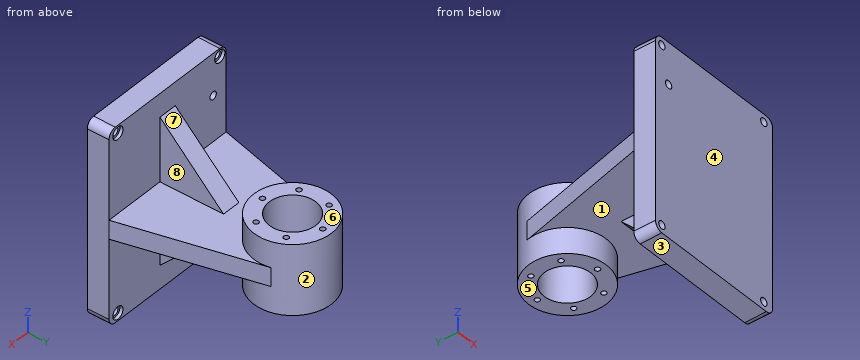
```python
from build123d import *

# Parameters (mm, degrees)
SKETCH_1_R                   = 25
SKETCH_1_R_2                 = 15
EXTRUDE_1_DEPTH              = 22.5
SKETCH_2_W                   = 92
SKETCH_2_H                   = 14
EXTRUDE_2_DEPTH              = 62
EXTRUDE_3_DEPTH              = 6
RIB_1_REACH                  = 123.639
SKETCH_5_WALL_W              = 303.26037525
SKETCH_5_WALL_H              = 12
FILLET_1_R                   = 5
HOLE_WIZARD_M4_2_D           = 5
HOLE_WIZARD_M4_2_CBORE_D     = 8
HOLE_WIZARD_M4_2_CBORE_DEPTH = 2
PATTERN_LINEAR_1_COUNT       = 2
PATTERN_LINEAR_1_PITCH       = 80
PATTERN_LINEAR_1_COUNT_DIR2  = 2
PATTERN_LINEAR_1_PITCH_DIR2  = 114
HOLE_WIZARD_M6_1_D           = 5
PATTERN_CIRCULAR_1_COUNT     = 6


with BuildPart() as part:
    # Sketch 1 → Extrude 1 (new, symmetric)
    with BuildSketch(Plane.XY):
        with Locations(Location((0, 0.57540869, 0), (0, 0, 180))):
            Circle(SKETCH_1_R)
        with Locations(Location((0, 0.57540869, 0), (0, 0, 180))):
            Circle(SKETCH_1_R_2, mode=Mode.SUBTRACT)
    extrude(amount=EXTRUDE_1_DEPTH, both=True)



with BuildPart() as body_2:
    # Sketch 2 → Extrude 2 (new, symmetric)
    with BuildSketch(Plane.XY):
        with Locations((0, -87)):
            Rectangle(SKETCH_2_W, SKETCH_2_H)
    extrude(amount=EXTRUDE_2_DEPTH, both=True)


with BuildPart() as part_1:
    add(part.part)

    add(body_2.part)  # Extrude 3 merges body 2
    # Sketch 4 → Extrude 3 (add, symmetric)
    with BuildSketch(Plane.XY):
        with BuildLine():
            Line((-24.247840613, 6.661641155), (-46, -80))
            Line((-46, -80), (46, -80))
            Line((46, -80), (24.247840613, 6.661641155))
            ThreePointArc((24.247840613, 6.661641155), (0, -24.42459131), (-24.247840613, 6.661641155))
        make_face()
    extrude(amount=EXTRUDE_3_DEPTH, both=True)

    # Sketch 5 wall → Rib 1 (add, up to next)
    with BuildSketch(Plane(origin=(0, -59.5, 26.5), x_dir=(0, 0.707106781187, -0.707106781187), z_dir=(0, 0.707106781187, 0.707106781187)), mode=Mode.PRIVATE) as rib_1_sk1:
        Rectangle(SKETCH_5_WALL_W, SKETCH_5_WALL_H)
    rib_1_tool1 = extrude(rib_1_sk1.sketch, amount=-RIB_1_REACH, mode=Mode.PRIVATE) - part_1.part
    rib_1 = rib_1_tool1.solids().sort_by_distance((0, -59.5, 26.5))[0]
    add(rib_1)

    # Mirror 1: Rib 1 across plane
    add(rib_1.mirror(Plane.XY))

    # Fillet 1
    fillet_1_edges = [part_1.edges().sort_by_distance(p)[0] for p in [
        (-46, -87, -62),
        (46, -87, 62),
        (-46, -87, 62),
        (46, -87, -62),
    ]]
    fillet(fillet_1_edges, radius=FILLET_1_R)

    # Hole Wizard M4 _ _ _ _ _2 (through all)
    with Locations(Plane(origin=(-41, -80, 57), x_dir=(0, 0, 1), z_dir=(0, 1, 0))):
        with Locations((0, 0)):
            hole_wizard_m4_2 = CounterBoreHole(HOLE_WIZARD_M4_2_D / 2, HOLE_WIZARD_M4_2_CBORE_D / 2, HOLE_WIZARD_M4_2_CBORE_DEPTH)

    # Pattern Linear 1: Hole Wizard M4 _ _ _ _ _2 2 × 2
    with Locations(*[(i * PATTERN_LINEAR_1_PITCH, 0, -j * PATTERN_LINEAR_1_PITCH_DIR2) for i in range(PATTERN_LINEAR_1_COUNT) for j in range(PATTERN_LINEAR_1_COUNT_DIR2) if (i, j) != (0, 0)]):
        add(hole_wizard_m4_2, mode=Mode.SUBTRACT)

    # Hole Wizard M6 _ _1 (through all)
    with Locations(Plane(origin=(-35.723311544, -80, 35.243458723), x_dir=(0, 0, 1), z_dir=(0, 1, 0))):
        with Locations((0, 0)):
            Hole(HOLE_WIZARD_M6_1_D / 2)

    # Sketch 21 → Hole Wizard M4 _ _1 (revolve, cut)
    with BuildSketch(Plane(origin=(0, 20, 22.5), x_dir=(0, -1, 0), z_dir=(1, 0, 0))):
        Polygon((0, 0), (0, 12.491420021), (1.65, 11.5), (1.65, 0), align=None)
    hole_wizard_m4_1 = revolve(axis=Axis((0, 20, 28.85), (0, 0, -1)), mode=Mode.SUBTRACT)

    # Pattern Circular 1: Hole Wizard M4 _ _1 ×6 about axis
    pattern_circular_1_axis = Axis((0, 0.57540869, 0), (0, 0, 1))
    for i in range(1, PATTERN_CIRCULAR_1_COUNT):
        add(hole_wizard_m4_1.rotate(pattern_circular_1_axis, i * 360 / PATTERN_CIRCULAR_1_COUNT), mode=Mode.SUBTRACT)

    # Mirror 2: Hole Wizard M4 _ _1 across plane
    add(hole_wizard_m4_1.mirror(Plane.XY), mode=Mode.SUBTRACT)

    # Mirror 2 copy 1 sketch → Mirror 2 copy 1 (revolve, cut)
    with BuildSketch(Plane(origin=(-16.822189532, 10.287704345, -22.5), x_dir=(0.8660254037844386, -0.5000000000000001, 0), z_dir=(0.5000000000000001, 0.8660254037844386, 0))):
        Polygon((0, 0), (0, -12.491420021), (1.65, -11.5), (1.65, 0), align=None)
    revolve(axis=Axis((-16.822189532, 10.287704345, -28.85), (0, 0, -1)), mode=Mode.SUBTRACT)

    # Mirror 2 copy 2 sketch → Mirror 2 copy 2 (revolve, cut)
    with BuildSketch(Plane(origin=(-16.822189532, -9.136886965, -22.5), x_dir=(0.8660254037844387, 0.4999999999999998, 0), z_dir=(-0.4999999999999998, 0.8660254037844387, 0))):
        Polygon((0, 0), (0, -12.491420021), (1.65, -11.5), (1.65, 0), align=None)
    revolve(axis=Axis((-16.822189532, -9.136886965, -28.85), (0, 0, -1)), mode=Mode.SUBTRACT)

    # Mirror 2 copy 3 sketch → Mirror 2 copy 3 (revolve, cut)
    with BuildSketch(Plane(origin=(0, -18.849182619, -22.5), x_dir=(0, 1, 0), z_dir=(-1, 0, 0))):
        Polygon((0, 0), (0, -12.491420021), (1.65, -11.5), (1.65, 0), align=None)
    revolve(axis=Axis((0, -18.849182619, -28.85), (0, 0, -1)), mode=Mode.SUBTRACT)

    # Mirror 2 copy 4 sketch → Mirror 2 copy 4 (revolve, cut)
    with BuildSketch(Plane(origin=(16.822189532, -9.136886965, -22.5), x_dir=(-0.8660254037844384, 0.5000000000000004, 0), z_dir=(-0.5000000000000004, -0.8660254037844384, 0))):
        Polygon((0, 0), (0, -12.491420021), (1.65, -11.5), (1.65, 0), align=None)
    revolve(axis=Axis((16.822189532, -9.136886965, -28.85), (0, 0, -1)), mode=Mode.SUBTRACT)

    # Mirror 2 copy 5 sketch → Mirror 2 copy 5 (revolve, cut)
    with BuildSketch(Plane(origin=(16.822189532, 10.287704345, -22.5), x_dir=(-0.8660254037844386, -0.5000000000000001, 0), z_dir=(0.5000000000000001, -0.8660254037844386, 0))):
        Polygon((0, 0), (0, -12.491420021), (1.65, -11.5), (1.65, 0), align=None)
    revolve(axis=Axis((16.822189532, 10.287704345, -28.85), (0, 0, -1)), mode=Mode.SUBTRACT)


solid = part_1.part
```
The model under review builds one solid part; all positions refer to its coordinate system, in mm. Face numbers are marked on the shaded views. A direction names the side the tool comes from. Round coordinates to 2 decimals unless told otherwise and drop trailing zeros. Loops run counter-clockwise (first coordinate to the right, second up) from the corner with the lowest first, then second, coordinate; pieces in that order, holes last. Notation, with made-up numbers: (59.5, -13.75) -> (85.5, -13.75) arc R8 cw to (85.5, -9.75) -> close; hole circle Ø8 at (71.25, 10). An arc over 180 degrees is marked (long way). Answer in a Markdown table with one row per item.
1) Consider section B-B, the plane z = 3.5. Write out the cut boundary in (x, y).
Taken from the geometry:
| item | result |
|---|---|
| outline | (-46, -94) -> (46, -94) -> (46, -80) -> (24.25, 6.66) arc R25 ccw to (-24.25, 6.66) -> (-46, -80) -> close; hole circle Ø30 at (0, 0.58) |
2) Consider section A-A, the plane z = -18. Count the separate pieces of the cut face and the enclosed holes in it, plus the area to 3 significant figures.
Taken from the geometry:
| item | result |
|---|---|
| separate pieces | 2 |
| enclosed holes | 7 |
| area | 2,840 mm² |
3) Consider section C-C, the plane y = -64. Write out the cut boundary in (x, z), plus the area to 3 significant figures.
Taken from the geometry:
| item | result |
|---|---|
| outline | (-41.98, -6) -> (-6, -6) -> (-6, -31) -> (6, -31) -> (6, -6) -> (41.98, -6) -> (41.98, 6) -> (6, 6) -> (6, 31) -> (-6, 31) -> (-6, 6) -> (-41.98, 6) -> close |
| area | 1,610 mm² |
4) Tool access review of the marked faces 5, 6, 7 and 8: name each direction out of +Z, -Z, +X, -X, +Y, -Y from which nothing blocks a thin tool from reaching the whole face with its end or side.
Taken from the geometry:
| item | result |
|---|---|
| face 5 | -Z, +X, -X, +Y |
| face 6 | +Z, +X, -X, +Y |
| face 7 | +Z, +X, -X |
| face 8 | +Z, +X |
5) Wall thickness on line 1 along Y through (x, z) = (0, 4); line 2 along Z through (x, y) = (-21, 11.5); line 3 along Y through (x, z) = (-37.5, -21.5): over which ranges is each line inside the solid? List them lowest first.
Taken from the geometry:
| item | result |
|---|---|
| line 1 | y = -94 to -14.42, 15.58 to 25.58 |
| line 2 | z = -22.5 to 22.5 |
| line 3 | y = -94 to -80 |
6) Draft analysis for pull direction Y (two halves, no side actions). For the marked faces 1, 2, 3 and 4, state which applies: pulls with the +Y half, pulls with the -Y half, needs draft (parallel to the pull), parting line crosses it, or undercut.
Taken from the geometry:
| item | result |
|---|---|
| face 1 | undercut |
| face 2 | undercut |
| face 3 | needs draft |
| face 4 | pulls with the -Y half |
7) For pin 1 Ø3 at (x, y) = (35, -23.5) entering from -Z; pin 2 Ø4 at (x, y) = (-16.82, 10.29) entering from -Z; pin 3 Ø1 at (y, z) = (-23, 16.5) entering from +X; pin 4 Ø4 at (x, z) = (-39.5, -57.5) entering from +Y, all flat-tipped, find the tip position at first contact; note any pin that passes through.
Taken from the geometry:
| item | result |
|---|---|
| pin 1 | passes through |
| pin 2 | stops at z = -22.5 |
| pin 3 | stops at x = 9.62 |
| pin 4 | stops at y = -82 |
